The listing builds one solid part. Answer for the finished solid, in the listing's coordinates (mm). A direction names the side the tool comes from. Coordinates: 2 decimals unless noted, no trailing zeros. Write each loop counter-clockwise with the first axis right and the second up, starting at its lowest first coordinate (ties: lowest second). Pieces come first, ordered by that corner, then holes.
from build123d import *

# Parameters (mm, degrees)
SKETCH1_W           = 14
SKETCH1_H           = 25
SKETCH1_R           = 1.55
BOSS_EXTRUDE1_DEPTH = 3
BOSS_EXTRUDE2_DEPTH = 20.5
SKETCH4_R           = 1.575
CUT_EXTRUDE1_DEPTH  = 38.057387927
CUT_EXTRUDE2_DEPTH  = 20.5
BOSS_EXTRUDE3_DEPTH = 2


with BuildPart() as part:
    # Sketch1 → Boss-Extrude1 (new body)
    with BuildSketch(Plane.XY):
        with Locations((7, 12.5)):
            Rectangle(SKETCH1_W, SKETCH1_H)
        with Locations((8, 19)):
            Circle(SKETCH1_R, mode=Mode.SUBTRACT)
        with Locations((8, 9)):
            Circle(SKETCH1_R, mode=Mode.SUBTRACT)
    extrude(amount=BOSS_EXTRUDE1_DEPTH)

    # Sketch3 → Boss-Extrude2 (add)
    with BuildSketch(Plane.XY.offset(3)):
        Polygon((0, 0), (0, 25), (14, 25), (14, 23), (2, 23), (2, 0), align=None)
    extrude(amount=BOSS_EXTRUDE2_DEPTH)

    # Sketch4 → Cut-Extrude1 (cut, through all)
    with BuildSketch(Plane.ZY):
        with Locations(Location((11.75, 15, 0), (0, 0, 270))):
            Circle(SKETCH4_R)
        with Locations(Location((11.75, 7, 0), (0, 0, 270))):
            Circle(SKETCH4_R)
    extrude(amount=-CUT_EXTRUDE1_DEPTH, mode=Mode.SUBTRACT)

    # Sketch5 → Cut-Extrude2 (cut)
    with BuildSketch(Plane(origin=(0, 23, 0), x_dir=(-1, 0, 0), z_dir=(0, -1, 0))):
        Polygon((-14, -3), (-2, -23.5), (-14, -23.5), align=None)
    extrude(amount=-CUT_EXTRUDE2_DEPTH, mode=Mode.SUBTRACT)

    # Sketch6 → Boss-Extrude3 (add)
    with BuildSketch(Plane(origin=(0, 0, 0), x_dir=(-1, 0, 0), z_dir=(0, -1, 0))):
        Polygon((-14, 0), (-14, -3), (-2, -23.5), (0, -23.5), (0, 0), align=None)
    extrude(amount=BOSS_EXTRUDE3_DEPTH)


solid = part.part
Q1. The part is cut by section B-B, the plane x = 8. Write down the section's boundary in (y, z).
Answers below:
outline: (-2, 0) - (7.45, 0) - (7.45, 3) - (0, 3) - (0, 13.25) - (-2, 13.25) - close; (10.55, 0) - (17.45, 0) - (17.45, 3) - (10.55, 3) - close; (20.55, 0) - (25, 0) - (25, 13.25) - (23, 13.25) - (23, 3) - (20.55, 3) - close
Q2. Determine the mould class of faces 3 (the face through (8, 12, 3)), 4 (the face through (6, -2, 9)), 5 (the face through (0.986, 8.573, 11.819)) for opening direction Z: released by +Z, released by -Z, zero draft, split by the parting line, or undercut.
Answers below:
face 3: released by +Z
face 4: zero draft
face 5: undercut
Q3. Which of the six approach directions +Z, -Z, +X, -X, +Y, -Y give full straight-line access (tool end or side, diameter ignored) to faces 1 (the face through (8.08, -0.99, 13.11)), 2 (the face through (2, 12, 13))?
Answers below:
face 1: +Z, +X, +Y, -Y
face 2: +Z, +X
Q4. Find the intervals of material crossed by probe 1 along Y at (x, z) = (8, 1); probe 2 along Y at (x, z) = (8.25, 9); probe 3 along Z at (x, y) = (1.65, 15) (3 decimals), in increasing order.
Answers below:
probe 1: y = -2 to 7.45, 10.55 to 17.45, 20.55 to 25
probe 2: y = -2 to 0, 23 to 25
probe 3: z = 0 to 10.175, 13.325 to 23.5
Q5. The part is cut by section D-D, the plane z = 17. Write down the section's boundary in (x, y), then the cut area to 3 significant figures.
Answers below:
outline: (0, -2) - (5.8, -2) - (5.8, 0) - (2, 0) - (2, 23) - (5.8, 23) - (5.8, 25) - (0, 25) - close
area: 69.2 mm2
Q6. Given pin 1 (5 mm diameter, centred on y = 7, z = 11.75, fed in from +X); pin 2 (4 mm diameter, centred on x = 8, y = 19, fed in from +Z); pin 3 (1.9 mm diameter, centred on y = 15, z = 11.75, fed in from +X), each flat-ended and moving along its own axis, determine where each tip first touches the part or whether it passes through.
Answers below:
pin 1: stops at x = 2
pin 2: stops at z = 3
pin 3: passes through
Q7. The part is cut by section C-C, the plane z = 13. Write down the section's boundary in (x, y).
Answers below:
outline: (0, -2) - (8.15, -2) - (8.15, 0) - (2, 0) - (2, 6.04) - (0, 6.04) - close; (0, 7.96) - (2, 7.96) - (2, 14.04) - (0, 14.04) - close; (0, 15.96) - (2, 15.96) - (2, 23) - (8.15, 23) - (8.15, 25) - (0, 25) - close
Q8. The part is cut by section A-A, the plane y = 7. Write down the section's boundary in (x, z) (3 decimals), then the cut area to 3 significant figures.
Answers below:
outline: (0, 0) - (14, 0) - (14, 3) - (2, 3) - (2, 10.175) - (0, 10.175) - close; (0, 13.325) - (2, 13.325) - (2, 23.5) - (0, 23.5) - close
area: 76.7 mm2
